For this review, take the finished solid that the model builds, in its own axes (mm). Face numbers are marked on the shaded views. A direction names the side the tool comes from. Give positions to 0.01 mm unless a question says otherwise; leave off trailing zeros. Order: outer loops, then holes, each group sorted by start corner. A loop starts at its lowest first (then second) coordinate and runs counter-clockwise, first axis right, second up. Notation, with made-up numbers: (51.25, 67.25) - (91.25, 67.25) arc R17 cw to (91.25, 90.25) - close; hole circle Ø11 at (-19, -6). An arc over 180 degrees is marked (long way). One line per item, written item: value.
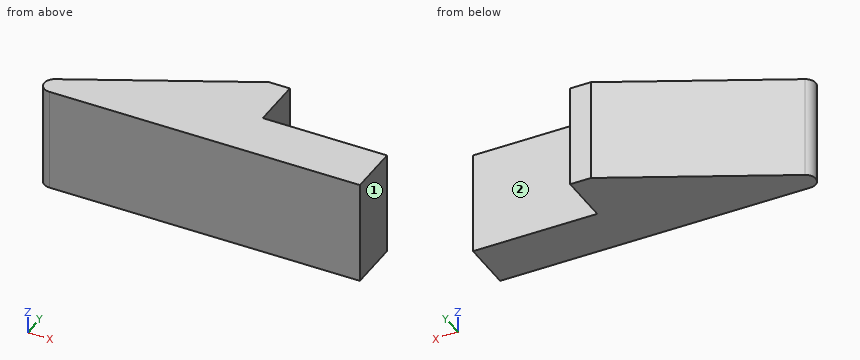
```python
from build123d import *

# Parameters (mm, degrees)
BASE_EXTRUDE_DEPTH = 5


with BuildPart() as part:
    # Sketch1 → Base-Extrude (new body, symmetric)
    with BuildSketch(Plane.XY):
        with BuildLine():
            Line((-0.442055564, 1.896987669), (16, 10))
            Line((16, 10), (18, 10))
            Line((18, 10), (18, 5))
            Line((18, 5), (30, 5))
            Line((30, 5), (30, 0))
            Line((30, 0), (0, 0))
            ThreePointArc((0, 0), (-0.973906481, 0.773050302), (-0.442055564, 1.896987669))
        make_face()
    extrude(amount=BASE_EXTRUDE_DEPTH, both=True)


solid = part.part
```
(1) Wall thickness on line 1 (Y direction, x = 21.5, z = -3.75); line 2 (Y direction, x = 11.5, z = 2.75); line 3 (X direction, y = 4, z = -1.5): over which ranges is each line inside the solid? List them lowest first. Write a range as from..to.
Answers below:
line 1: y = 0..5
line 2: y = 0..7.78
line 3: x = 3.83..30
(2) Take a section at C-C (y = 7.75). Write out the cut boundary in (x, z).
Answers below:
outline: (11.43, -5) - (18, -5) - (18, 5) - (11.43, 5) - close
(3) Machinability: for the marked faces 1 and 2, which of the approach directions +Z, -Z, +X, -X, +Y, -Y give a long, thin tool a straight path to every point of the face, cutting with its end or side? Answer none if there is none.
Answers below:
face 1: +Z, -Z, +X, +Y, -Y
face 2: +Z, -Z, +X, +Y
(4) Take a section at B-B (x = 28). Write out the cut boundary in (y, z).
Answers below:
outline: (0, -5) - (5, -5) - (5, 5) - (0, 5) - close
(5) Take a section at A-A (z = 2.25). Write out the cut boundary in (x, y), then the cut area to 3 significant figures.
Answers below:
outline: (-0.44, 1.9) arc R1 ccw to (0, 0) - (30, 0) - (30, 5) - (18, 5) - (18, 10) - (16, 10) - close
area: 179 mm^2
(6) For P1, Ø4, axis at x = 15, z = -2.5, coming from the -Y side; P2, Ø1.5, axis at x = 23, z = -2, coming from the +Y side; P3, Ø1.5, axis at x = 9, z = 2, coming from the +Y side; P4, Ø2.5, axis at y = 8.5, z = 0.5, coming from the +X side, all flat-tipped, find the tip position at first contact; note any pin that passes through.
Answers below:
P1: stops at y = 0
P2: stops at y = 5
P3: stops at y = 6.92
P4: stops at x = 18
